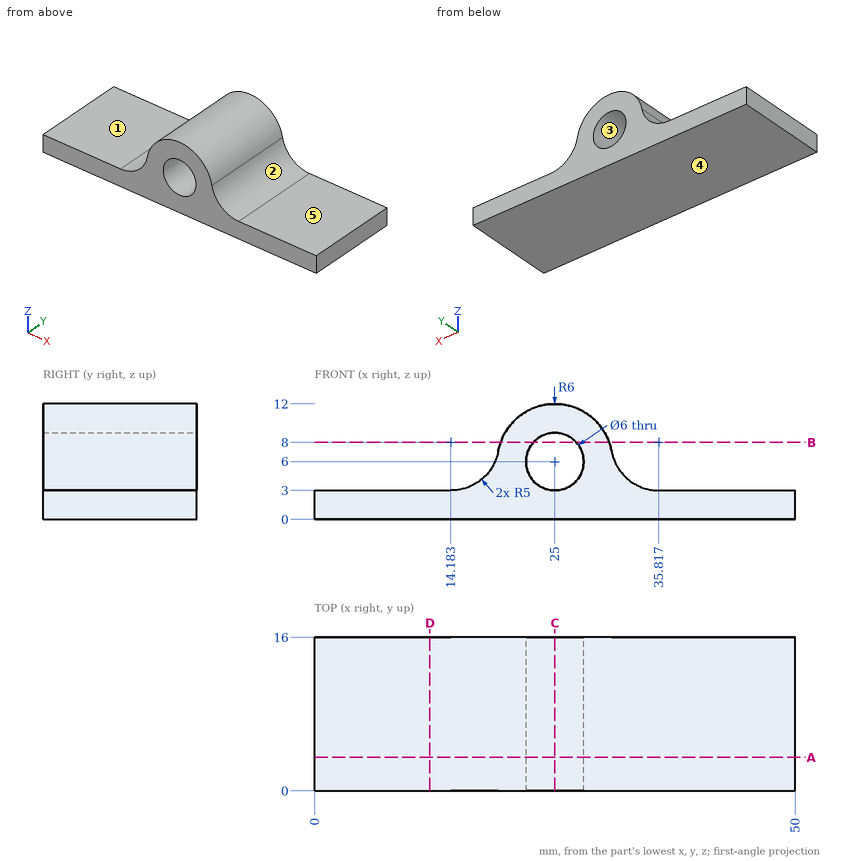
Geometry: see drawing. Coordinates: mm, zero at the bounding-box minimum. A direction names the side the tool comes from. Round coordinates to 2 decimals unless told otherwise and drop trailing zeros. Order: outer loops, then holes, each group sorted by start corner. A loop starts at its lowest first (then second) coordinate and runs counter-clockwise, first axis right, second up. Notation, with made-up numbers: (71.5, 54) - (110.5, 54) arc R20 ccw to (110.5, 79) - close; hole circle Ø1 at (-5.5, 22). An arc over 180 degrees is marked (long way). Use a Markdown table: item, result. Add a question column.
1. Section query A-A (y = 3.5). Return the cut outline in (x, z).
2. Line query: probe 1 along Z at (x, y) = (25, 4.25); probe 2 along Z at (x, y) = (43, 9.75); probe 3 along Z at (x, y) = (27, 1.5) (1 decimal). Output: solid intervals per line, ascending.
3. First-contact query: pin 1 (5 mm diameter, centred on x = 25, z = 6, fed in from -Y); pin 2 (1 mm diameter, centred on x = 11.5, y = 7, fed in from +Z); pin 3 (6 mm diameter, centred on y = 2.5, z = 10.5, fed in from -X); pin 4 (1 mm diameter, centred on y = 11.5, z = 4.5, fed in from -X) (1 decimal). Flat tips, straight axial feed; report the tip coordinate or a pass-through.
4. Section query B-B (z = 8). Return the cut outline in (x, y).
5. Mould query, pull axis Z, two halves, no side actions, for the marked faces 3, 4 and 5. Classes: +Z half, -Z half, draft (parallel to the pull), parting line (faces both ways), or undercut.
6. Section query D-D (x = 12). Return the cut outline in (y, z), then the cut area to 3 significant figures.
7. Set-up query: the marked faces 1 and 2. Return all of +Z, -Z, +X, -X, +Y, -Y with unobstructed straight access to the full face (end or side cutting, diameter ignored); none if empty.
8. Section query C-C (x = 25). Return the cut outline in (y, z).
Derived:
| question | item | result |
|---|---|---|
| 1 | outline | (0, 0) - (50, 0) - (50, 3) - (35.82, 3) arc R5 cw to (30.9, 7.09) arc R6 ccw to (19.1, 7.09) arc R5 cw to (14.18, 3) - (0, 3) - close; hole circle Ø6 at (25, 6) |
| 2 | probe 1 | 0 to 3, 9 to 12 |
| 2 | probe 2 | 0 to 3 |
| 2 | probe 3 | 0 to 3.8, 8.2 to 11.7 |
| 3 | pin 1 | through |
| 3 | pin 2 | z = 3 |
| 3 | pin 3 | x = 19.19 |
| 3 | pin 4 | x = 17.2 |
| 4 | outline | (19.34, 0) - (22.76, 0) - (22.76, 16) - (19.34, 16) - close; (27.24, 0) - (30.66, 0) - (30.66, 16) - (27.24, 16) - close |
| 5 | face 3 | undercut |
| 5 | face 4 | -Z half |
| 5 | face 5 | +Z half |
| 6 | outline | (0, 0) - (16, 0) - (16, 3) - (0, 3) - close |
| 6 | area | 48.0 mm2 |
| 7 | face 1 | +Z, -X, +Y, -Y |
| 7 | face 2 | +Z, +X, +Y, -Y |
| 8 | outline | (0, 0) - (16, 0) - (16, 3) - (0, 3) - close; (0, 9) - (16, 9) - (16, 12) - (0, 12) - close |
